Check sheet for the modelled part. Datum: model origin and axes. Units: mm. Coordinates: 2 decimals unless noted, no trailing zeros. Write each loop counter-clockwise with the first axis right and the second up, starting at its lowest first coordinate (ties: lowest second). Pieces come first, ordered by that corner, then holes. Notation, with made-up numbers: M 81.5,54 L 86.5,54 A32 ccw 86.5,83 Z; hole C 65.5,16 d7. An arc over 180 degrees is marked long. Answer as CSV lines item,"result".
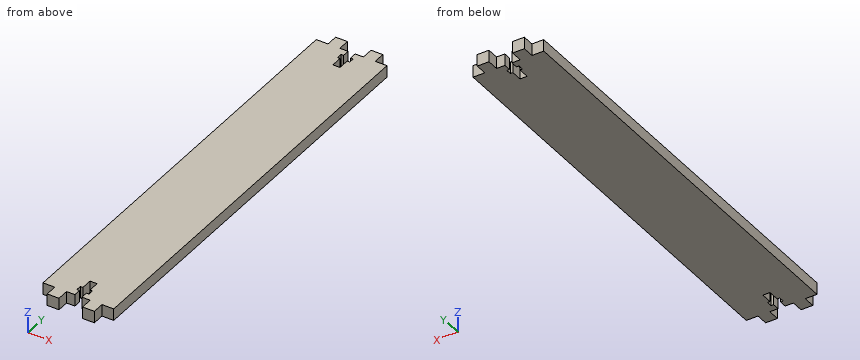
from build123d import *

# Parameters (mm, degrees)
BOSS_EXTRU_1_DEPTH = 5


with BuildPart() as part:
    # Esquisse1 → Boss.-Extru.1 (new body)
    with BuildSketch(Plane.XY):
        Polygon((-15, 185), (-15, 95), (15, 95), (15, 185), (10, 185), (10, 190), (5, 190), (5, 185), (1.5, 185), (1.5, 182), (2.6, 182), (2.6, 179.7), (1.5, 179.7), (1.5, 175), (-1.5, 175), (-1.5, 179.7), (-2.6, 179.7), (-2.6, 182), (-1.5, 182), (-1.5, 185), (-5, 185), (-5, 190), (-10, 190), (-10, 185), align=None)
        Polygon((-15, 5), (-10, 5), (-10, 0), (-5, 0), (-5, 5), (-1.5, 5), (-1.5, 8), (-2.6, 8), (-2.6, 10.3), (-1.5, 10.3), (-1.5, 15), (1.5, 15), (1.5, 10.3), (2.6, 10.3), (2.6, 8), (1.5, 8), (1.5, 5), (5, 5), (5, 0), (10, 0), (10, 5), (15, 5), (15, 95), (-15, 95), align=None)
    extrude(amount=BOSS_EXTRU_1_DEPTH)


solid = part.part
1) Thickness scan on line 1 along X through (y, z) = (179, 4.4); line 2 along Y through (x, z) = (12.5, 1.25); line 3 along Y through (x, z) = (1, 1.6). Record the ranges inside material, lowest first.
Answer key:
line 1,"x = -15 to -1.5, 1.5 to 15"
line 2,"y = 5 to 185"
line 3,"y = 15 to 175"
2) Section check A-A, the plane x = -12.5. Record the boundary of the cut face in (y, z), plus the area to 3 significant figures.
Answer key:
outline,"M 5,0 L 185,0 L 185,5 L 5,5 Z"
area,"900 mm2"
3) Depth check by flat-ended pin: P1, Ø0.6, axis at x = 2, z = 3, coming from the +Y side; P2, Ø1.2, axis at x = -2, z = 3, coming from the -Y side; P3, Ø2.5, axis at y = 3, z = 2.5, coming from the +X side. Enter the tip coordinate at first touch or a pass-through.
Answer key:
P1,"stops at y = 185"
P2,"stops at y = 5"
P3,"stops at x = 10"
